The listing builds one solid part. Answer for the finished solid, in the listing's coordinates (mm). A direction names the side the tool comes from. Coordinates: 2 decimals unless noted, no trailing zeros. Loops run counter-clockwise (first coordinate to the right, second up) from the corner with the lowest first, then second, coordinate; pieces in that order, holes last. Notation, with made-up numbers: (39.5, -4.5) -> (75.5, -4.5) arc R12 ccw to (75.5, 6.5) -> close; hole circle Ø9 at (50, -6). An arc over 180 degrees is marked (long way). Answer in a Markdown table with one row per item.
```python
from build123d import *

# Parameters (mm, degrees)
SKETCH1_R           = 13
BOSS_EXTRUDE1_DEPTH = 6
SKETCH2_R           = 17.53
BOSS_EXTRUDE2_DEPTH = 15.3
SKETCH3_R           = 2.5
BOSS_EXTRUDE3_DEPTH = 15
CHAMFER1_SIZE       = 0.5
SKETCH4_R           = 7
CUT_EXTRUDE1_DEPTH  = 6


with BuildPart() as part:
    # Sketch1 → Boss-Extrude1 (new body)
    with BuildSketch(Plane(origin=(0, 0, 0), x_dir=(1, 0, 0), z_dir=(0, 1, 0))):
        Circle(SKETCH1_R)
    extrude(amount=BOSS_EXTRUDE1_DEPTH)

    # Sketch2 → Boss-Extrude2 (add)
    with BuildSketch(Plane(origin=(0, 6, 0), x_dir=(1, 0, 0), z_dir=(0, 1, 0))):
        Circle(SKETCH2_R)
    extrude(amount=BOSS_EXTRUDE2_DEPTH)

    # Sketch3 → Boss-Extrude3 (add)
    with BuildSketch(Plane(origin=(0, 21.3, 0), x_dir=(1, 0, 0), z_dir=(0, 1, 0))):
        Circle(SKETCH3_R)
    extrude(amount=BOSS_EXTRUDE3_DEPTH)

    # Chamfer1
    chamfer1_edges = [part.edges().sort_by_distance(p)[0] for p in [
        (-17.53, 21.3, 0),
    ]]
    chamfer(chamfer1_edges, length=CHAMFER1_SIZE)

    # Sketch4 → Cut-Extrude1 (cut)
    with BuildSketch(Plane.XZ):
        Circle(SKETCH4_R)
    extrude(amount=-CUT_EXTRUDE1_DEPTH, mode=Mode.SUBTRACT)


solid = part.part
```
Item 1: A tool of negligible diameter and unlimited length cuts with its end or side. For faces 4 (the face through (-12, 6, 6)), 5 (the face through (-0.54, 28.7, 2.44)), 6 (the face through (-2.28, 13.3, -17.38)), from which of +Z, -Z, +X, -X, +Y, -Y can it reach the whole face along a straight path? Write none if from no direction.
Findings below:
| item | result |
|---|---|
| face 4 | -Y |
| face 5 | +Y |
| face 6 | +Y, -Y |
Item 2: A cutting plane is placed at D-D, the plane y = 9.5. Determine the outline of the cut face in (x, z).
Findings below:
| item | result |
|---|---|
| outline | circle Ø35.06 at (0, 0) |
Item 3: Flat-ended cylindrical pins translate along their axes: pin 1 Ø10 at (x, z) = (-12.5, -6) entering from +Y; pin 2 Ø2 at (x, y) = (6, 12.5) entering from +Z; pin 3 Ø5 at (x, y) = (-3.5, 14.5) entering from -Z. Find the tip coordinate at first contact, or state that the pin passes through.
Findings below:
| item | result |
|---|---|
| pin 1 | stops at y = 21.3 |
| pin 2 | stops at z = 16.8 |
| pin 3 | stops at z = -17.5 |
Item 4: A cutting plane is placed at B-B, the plane x = 0. Determine the outline of the cut face in (y, z).
Findings below:
| item | result |
|---|---|
| outline | (0, -13) -> (6, -13) -> (6, -17.53) -> (20.8, -17.53) -> (21.3, -17.03) -> (21.3, -2.5) -> (36.3, -2.5) -> (36.3, 2.5) -> (21.3, 2.5) -> (21.3, 17.03) -> (20.8, 17.53) -> (6, 17.53) -> (6, 13) -> (0, 13) -> (0, 7) -> (6, 7) -> (6, -7) -> (0, -7) -> close |
Item 5: Determine the mould class of faces 1 (the face through (6.466, 2.958, -2.681)), 2 (the face through (0, 36.3, 0)), 3 (the face through (-10.316, 2.958, 7.91)) for opening direction X: +X half, -X half, draft (parallel to the pull), parting line (faces both ways), or undercut.
Findings below:
| item | result |
|---|---|
| face 1 | undercut |
| face 2 | draft |
| face 3 | parting line |
Item 6: Find the intervals of material crossed by probe 1 along Z at (x, y) = (0, 3.95); probe 2 along Y at (x, z) = (8.5, 3); probe 3 along Y at (x, z) = (-6, -0.5), in increasing order.
Findings below:
| item | result |
|---|---|
| probe 1 | z = -13 to -7, 7 to 13 |
| probe 2 | y = 0 to 21.3 |
| probe 3 | y = 6 to 21.3 |
Item 7: A cutting plane is placed at A-A, the plane z = 0. Determine the outline of the cut face in (x, y).
Findings below:
| item | result |
|---|---|
| outline | (-17.53, 6) -> (-13, 6) -> (-13, 0) -> (-7, 0) -> (-7, 6) -> (7, 6) -> (7, 0) -> (13, 0) -> (13, 6) -> (17.53, 6) -> (17.53, 20.8) -> (17.03, 21.3) -> (2.5, 21.3) -> (2.5, 36.3) -> (-2.5, 36.3) -> (-2.5, 21.3) -> (-17.03, 21.3) -> (-17.53, 20.8) -> close |
Item 8: A cutting plane is placed at C-C, the plane y = 25. Determine the outline of the cut face in (x, z).
Findings below:
| item | result |
|---|---|
| outline | circle Ø5 at (0, 0) |
